For this review, take the finished solid that the model builds, in its own axes (mm). Face numbers are marked on the shaded views. A direction names the side the tool comes from. Round coordinates to 2 decimals unless told otherwise and drop trailing zeros. Write each loop counter-clockwise with the first axis right and the second up, starting at its lowest first coordinate (ties: lowest second). Pieces come first, ordered by that corner, then holes. Notation, with made-up numbers: (-23, 39.25) -> (14, 39.25) arc R19 cw to (14, 49.25) -> close; hole circle Ø6 at (36.5, -25.75). An arc over 180 degrees is marked (long way). Answer in a Markdown table with one row per item.
from build123d import *

# Parameters (mm, degrees)
F0_R        = 1.45
F1_DEPTH    = 17.5
F2_R        = 2.9
F3_DEPTH    = 1.8
F4_W        = 1
F4_H        = 1
F5_DEPTH    = 1.5
F6_S5_R     = 1.45
F6_T6_DEPTH = 6


# Not quite as in the source:
# - a fillet or chamfer that OpenCascade refuses, or shapes differently, is made with other operations: its cross-section is extruded or revolved along the edge and cut away or added


with BuildPart() as f1:
    # F0 (on Top) → F1 (new body)
    with BuildSketch(Plane.XY):
        Circle(F0_R)
    extrude(amount=F1_DEPTH)

    # F2 (on Top) → F3 (join)
    with BuildSketch(Plane.XY):
        Circle(F2_R)
    extrude(amount=-F3_DEPTH)

    # F4 (on face) → F5 (cut)
    with BuildSketch(Plane(origin=(0, 0, -1.8), x_dir=(1, 0, 0), z_dir=(0, 0, -1))):
        with Locations((1, 0)):
            Rectangle(F4_W, F4_H)
        Rectangle(F4_W, F4_H)
        with Locations((0, 1)):
            Rectangle(F4_W, F4_H)
        with Locations((-1, 0)):
            Rectangle(F4_W, F4_H)
        with Locations((0, -1)):
            Rectangle(F4_W, F4_H)
    extrude(amount=-F5_DEPTH, mode=Mode.SUBTRACT)

    # F6: chamfer of 1.5 on 1 edges, made by hand


with BuildPart() as f6_tool2:
    # F6_s3 → F6_t4 (revolve)
    with BuildSketch(Plane.XZ):
        Polygon((2.9, -1.5), (1.4, 0), (2.9, 0), align=None)
    revolve(axis=Axis((0, 0, 0), (0, 0, 1)))

    # F6_s5 → F6_t6 (cut, symmetric)
    with BuildSketch(Plane.XY.offset(-0.7)):
        Circle(F6_S5_R)
    extrude(amount=F6_T6_DEPTH, both=True, mode=Mode.SUBTRACT)


with BuildPart() as f1_1:
    add(f1.part)

    # F6_t1: cut F6_tool2
    add(f6_tool2.part, mode=Mode.SUBTRACT)


solid = f1_1.part
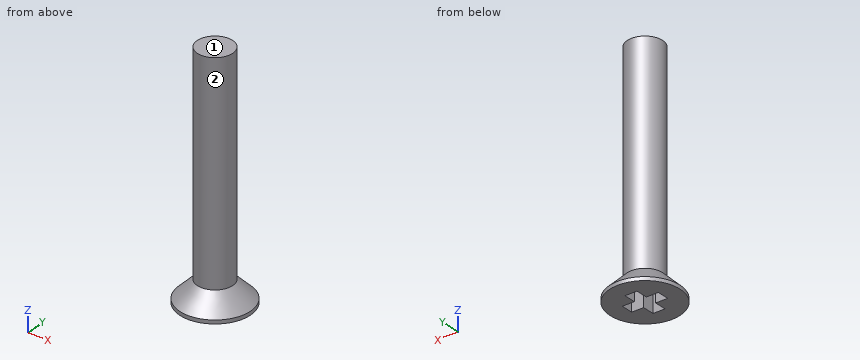
1) For the marked faces 1 and 2, list the 3-axis set-ups (+Z, -Z, +X, -X, +Y, -Y) from which the entire face can be reached by the end or side of a thin tool; tool diameter is ignored.
Solved:
| item | result |
|---|---|
| face 1 | +Z, +X, -X, +Y, -Y |
| face 2 | +Z |
2) For line 1 (Z direction, x = -0.1, y = 1.05); line 2 (Y direction, x = 0.1, z = 3.5); line 3 (Z direction, x = -1.3, y = -1.1), list the stretches that pass through material, from the lowest coordinate up. Write a range as [from, to].
Solved:
| item | result |
|---|---|
| line 1 | [-0.3, 17.5] |
| line 2 | [-1.45, 1.45] |
| line 3 | [-1.8, -0.3] |
3) Consider section C-C on z = 1. State the section outline as (x, y) points, then the cut area to 3 significant figures.
Solved:
| item | result |
|---|---|
| outline | circle Ø2.9 at (0, 0) |
| area | 6.61 mm² |
4) Clearance check with flat-ended pins moving along their axes: pin 1 Ø2 at (x, z) = (-0.5, 13.5) entering from +Y; pin 2 Ø0.8 at (y, z) = (1, -1) entering from +X; pin 3 Ø0.5 at (y, z) = (-1, -1.5) entering from -X; pin 4 Ø1.1 at (x, z) = (0, -1) entering from +Y. State where each tip first meets the part, or that it passes through.
Solved:
| item | result |
|---|---|
| pin 1 | y = 1.45 |
| pin 2 | x = 2.64 |
| pin 3 | x = -2.8 |
| pin 4 | y = 2.9 |
5) Consider section A-A on y = 0. State the section outline as (x, z) points.
Solved:
| item | result |
|---|---|
| outline | (-2.9, -1.8) -> (-1.5, -1.8) -> (-1.5, -0.3) -> (1.5, -0.3) -> (1.5, -1.8) -> (2.9, -1.8) -> (2.9, -1.5) -> (1.45, -0.05) -> (1.45, 17.5) -> (-1.45, 17.5) -> (-1.45, -0.05) -> (-2.9, -1.5) -> close |
